```python
from build123d import *

# Parameters (mm, degrees)
ESQUISSE1_R        = 3
BOSS_EXTRU_1_DEPTH = 10
ESQUISSE2_R        = 5
BOSS_EXTRU_3_DEPTH = 5
BOSS_EXTRU_4_START = 5
ESQUISSE3_R        = 5
BOSS_EXTRU_4_DEPTH = 5


with BuildPart() as part:
    # Esquisse1 → Boss.-Extru.1 (new body)
    with BuildSketch(Plane.XY):
        Circle(ESQUISSE1_R)
    extrude(amount=BOSS_EXTRU_1_DEPTH)

    # Esquisse2 → Boss.-Extru.3 (add)
    with BuildSketch(Plane.XY.offset(10)):
        Circle(ESQUISSE2_R)
    extrude(amount=BOSS_EXTRU_3_DEPTH)

    # Esquisse3 → Boss.-Extru.4 (add)
    with BuildSketch(Plane(origin=(0, 0, 0), x_dir=(-1, 0, 0), z_dir=(0, 0, -1)).offset(BOSS_EXTRU_4_START)):
        with Locations(Location((0, 0, 0), (0, 0, 180))):
            Circle(ESQUISSE3_R)
    extrude(amount=-BOSS_EXTRU_4_DEPTH)


solid = part.part
```
Model file for the job. Use its own axes, mm. A direction names the side the tool comes from. Coordinates: 2 decimals unless noted, no trailing zeros. Loops run counter-clockwise (first coordinate to the right, second up) from the corner with the lowest first, then second, coordinate; pieces in that order, holes last. Notation, with made-up numbers: (74.5, 21) -> (133.5, 21) arc R27 cw to (133.5, 53) -> close; hole circle Ø3 at (49.5, 13). An arc over 180 degrees is marked (long way). Answer as a JSON object with one key per item and string values.
Q1. Cut at D-D (z = 3.25). List the corners of the cut face in (x, y).
Report:
{"outline": "circle Ø6 at (0, 0)"}
Q2. Cut at A-A (y = 0). List the corners of the cut face in (x, z), and give its area (3 significant figures).
Report:
{"outline": "(-5, -5) -> (5, -5) -> (5, 0) -> (3, 0) -> (3, 10) -> (5, 10) -> (5, 15) -> (-5, 15) -> (-5, 10) -> (-3, 10) -> (-3, 0) -> (-5, 0) -> close", "area": "160 mm2"}
Q3. 3-axis set-ups, long thin cutter, end or side, ignore diameter. For faces 4 (the flat face through (-0.1, -3.3, 10)), 5 (the cylindrical face through (-5, 0, -3)): which of +Z, -Z, +X, -X, +Y, -Y reach the whole face in a straight line?
Report:
{"face 4": "none", "face 5": "+Z, -Z"}
Q4. Probe probe 1 along Z at (x, y) = (3.5, 1.25); probe 2 along Y at (x, z) = (-0.75, 14.25); probe 3 along Y at (x, z) = (-1.25, 13.5). List the from-to ranges inside material, lowest first.
Report:
{"probe 1": "z = -5 to 0, 10 to 15", "probe 2": "y = -4.94 to 4.94", "probe 3": "y = -4.84 to 4.84"}
Q5. Pull direction Z, two halves, no side cores. Call faces 1 (the cylindrical face through (-1.08, -4.88, 12.46)), 2 (the flat face through (0, 0, -5)), 3 (the cylindrical face through (-3, 0, 5)): released by +Z, released by -Z, zero draft, split by the parting line, or undercut.
Report:
{"face 1": "zero draft", "face 2": "released by -Z", "face 3": "undercut"}
Q6. Cut at B-B (x = 4). List the corners of the cut face in (y, z), and give its area (3 significant figures).
Report:
{"outline": "(-3, -5) -> (3, -5) -> (3, 0) -> (-3, 0) -> close; (-3, 10) -> (3, 10) -> (3, 15) -> (-3, 15) -> close", "area": "60.0 mm2"}
Q7. Flat gauge pins, fed straight in: P1, Ø1.5, axis at x = -2, z = 11, coming from the -Y side; P2, Ø1.5, axis at y = -3.5, z = 12, coming from the -X side; P3, Ø6, axis at x = 1.5, z = 5, coming from the -Y side; P4, Ø4, axis at x = 1.5, z = 12.5, coming from the +Y side. Where does each tip first touch, or does it go through?
Report:
{"P1": "stops at y = -4.84", "P2": "stops at x = -4.18", "P3": "stops at y = -3", "P4": "stops at y = 5"}
